Part model, mm, in its own coordinate system. Face numbers are marked on the shaded views. A direction names the side the tool comes from. Give positions to 0.01 mm unless a question says otherwise; leave off trailing zeros. Write each loop counter-clockwise with the first axis right and the second up, starting at its lowest first coordinate (ties: lowest second). Pieces come first, ordered by that corner, then holes. Notation, with made-up numbers: (6.25, 85.25) - (21.25, 85.25) arc R25 ccw to (21.25, 123.25) - close; hole circle Ø7 at (-33.5, 41). An arc over 180 degrees is marked (long way). Answer as a JSON object with one key per item and string values. Group by question number.
```python
from build123d import *

# Parameters (mm, degrees)
F0_W        = 85
F0_H        = 56
F1_DEPTH    = 1.6
F2_D        = 2.8
F3_W        = 50.8
F3_H        = 5.08
F4_DEPTH    = 2.54
F5_W        = 17.8862189412
F5_H        = 13.1
F6_DEPTH    = 14.8
F7_W        = 20.1875766277
F7_H        = 15.9
F8_DEPTH    = 13.5
F9_T1_DEPTH = 19.1
F9_T3_DEPTH = 10.35


# Not quite as in the source:
# - a fillet or chamfer that OpenCascade refuses, or shapes differently, is made with other operations: its cross-section is extruded or revolved along the edge and cut away or added


with BuildPart() as f1:
    # F0 (on Top) → F1 (new body)
    with BuildSketch(Plane.XY):
        Rectangle(F0_W, F0_H)
    extrude(amount=F1_DEPTH)

    # F2 (through all)
    with Locations(Plane(origin=(0, 0, 0), x_dir=(1, 0, 0), z_dir=(0, 0, -1))):
        with Locations((-39, -24.5), (19, -24.5), (19, 24.5), (-39, 24.5)):
            Hole(F2_D / 2)

    # F3 (on face) → F4 (join)
    with BuildSketch(Plane.XY.offset(1.6)):
        with Locations((-10.1, 24.5)):
            Rectangle(F3_W, F3_H)
    extrude(amount=F4_DEPTH)

    # F5 (on face) → F6 (join)
    with BuildSketch(Plane.XY.offset(1.6)):
        with Locations((35.6568905294, 18.95)):
            Rectangle(F5_W, F5_H)
        with Locations((35.6568905294, 0.95)):
            Rectangle(F5_W, F5_H)
    extrude(amount=F6_DEPTH)

    # F7 (on face) → F8 (join)
    with BuildSketch(Plane.XY.offset(1.6)):
        with Locations((34.5062116861, -17.75)):
            Rectangle(F7_W, F7_H)
    extrude(amount=F8_DEPTH)

    # F9: fillet of radius 3.5 on 4 edges, made by hand

    # F9_s2 → F9_t1 (cut)
    with BuildSketch(Plane.XY.offset(-8.75)):
        with BuildLine():
            ThreePointArc((-39, -28), (-41.4748737342, -26.9748737342), (-42.5, -24.5))
            Line((-42.5, -24.5), (-42.5, -28))
            Line((-42.5, -28), (-39, -28))
        make_face()
        with BuildLine():
            ThreePointArc((-42.5, 24.5), (-41.4748737342, 26.9748737342), (-39, 28))
            Line((-39, 28), (-42.5, 28))
            Line((-42.5, 28), (-42.5, 24.5))
        make_face()
    extrude(amount=F9_T1_DEPTH, mode=Mode.SUBTRACT)

    # F9_s4 → F9_t3 (cut)
    with BuildSketch(Plane.XY.offset(-8.75)):
        with BuildLine():
            ThreePointArc((39, -28), (41.4748737342, -26.9748737342), (42.5, -24.5))
            Line((42.5, -24.5), (42.5, -28))
            Line((42.5, -28), (39, -28))
        make_face()
        with BuildLine():
            ThreePointArc((42.5, 24.5), (41.4748737342, 26.9748737342), (39, 28))
            Line((39, 28), (42.5, 28))
            Line((42.5, 28), (42.5, 24.5))
        make_face()
    extrude(amount=F9_T3_DEPTH, mode=Mode.SUBTRACT)


solid = f1.part
```
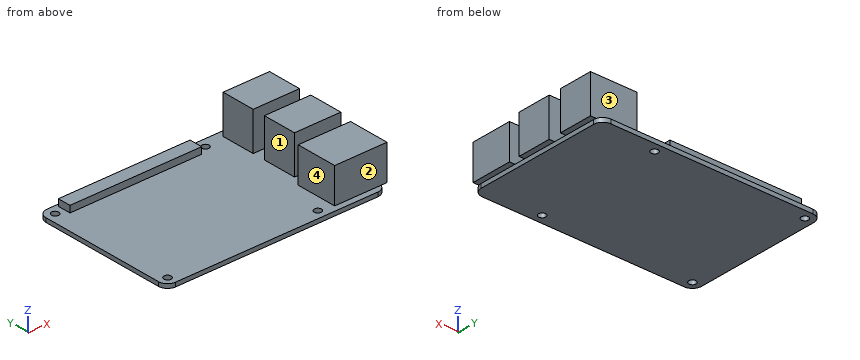
1) Saw through at A-A (z = 11.75). List the corners of the cut face in (x, y), and give its area (3 significant figures).
2) Drop flat-ended pins along their axis: P1, Ø1.1, axis at x = 43.5, y = 16, coming from the -Z side; P2, Ø2, axis at x = 25, z = 5, coming from the -Y side; P3, Ø3, axis at y = 25.5, z = 2.5, coming from the -X side; P4, Ø1.3, axis at y = -7.5, z = 0.5, coming from the +X side. Give the stop position or say it passes through.
3) Drill centre lines: line 1 along Y through (x, z) = (-39, 0.35); line 2 along X through (y, z) = (24.5, 0.7); line 3 along Y through (x, z) = (33.5, 8.5). Where is each one in solid material? Low to high. Write a range as from..to.
4) Saw through at D-D (x = 31.5). List the corners of the cut face in (y, z).
5) Saw through at C-C (y = -3). List the corners of the cut face in (x, z).
6) Which spindle directions (+Z, -Z, +X, -X, +Y, -Y) get a long thin tool onto all of the face, cutting with end or side? Do the marked faces 1, 2, 3 and 4. Say none if no direction does.
7) Saw through at B-B (x = -12). List the corners of the cut face in (y, z).
Checks:
{
 "1": {"outline": "(24.41, -25.7) - (44.6, -25.7) - (44.6, -9.8) - (24.41, -9.8) - close; (26.71, -5.6) - (44.6, -5.6) - (44.6, 7.5) - (26.71, 7.5) - close; (26.71, 12.4) - (44.6, 12.4) - (44.6, 25.5) - (26.71, 25.5) - close", "area": "790 mm2"},
 "2": {"P1": "z = 1.6", "P2": "y = -25.7", "P3": "x = -42.5", "P4": "x = 42.5"},
 "3": {"line 1": "-28..-25.9, -23.1..23.1, 25.9..28", "line 2": "-42.5..-40.4, -37.6..17.6, 20.4..42.5", "line 3": "-25.7..-9.8, -5.6..7.5, 12.4..25.5"},
 "4": {"outline": "(-28, 0) - (28, 0) - (28, 1.6) - (25.5, 1.6) - (25.5, 16.4) - (12.4, 16.4) - (12.4, 1.6) - (7.5, 1.6) - (7.5, 16.4) - (-5.6, 16.4) - (-5.6, 1.6) - (-9.8, 1.6) - (-9.8, 15.1) - (-25.7, 15.1) - (-25.7, 1.6) - (-28, 1.6) - close"},
 "5": {"outline": "(-42.5, 0) - (42.5, 0) - (42.5, 1.6) - (44.6, 1.6) - (44.6, 16.4) - (26.71, 16.4) - (26.71, 1.6) - (-42.5, 1.6) - close"},
 "6": {"face 1": "+Z, -X, +Y", "face 2": "+Z, +X, -X, -Y", "face 3": "+Z, +X, +Y", "face 4": "+Z, -X, +Y, -Y"},
 "7": {"outline": "(-28, 0) - (28, 0) - (28, 1.6) - (27.04, 1.6) - (27.04, 4.14) - (21.96, 4.14) - (21.96, 1.6) - (-28, 1.6) - close"}
}
